CAD build for the part. Positions are in the model's coordinates, mm. Face numbers are marked on the shaded views. A direction names the side the tool comes from. Give positions to 0.01 mm unless a question says otherwise; leave off trailing zeros. Loops run counter-clockwise (first coordinate to the right, second up) from the corner with the lowest first, then second, coordinate; pieces in that order, holes last.
Item 1: Saw through at B-B on x = 27.5. Give the cut face in (y, z).
Item 2: Drop flat-ended pins along their axis: P1, Ø1, axis at x = 22, y = -55, coming from the +Z side; P2, Ø15.5, axis at y = -67.5, z = 73, coming from the -X side; P3, Ø17.5, axis at x = 43.5, y = -8.5, coming from the +Z side. Give the stop position or say it passes through.
Item 3: Which spindle directions (+Z, -Z, +X, -X, +Y, -Y) get a long thin tool onto all of the face, cutting with end or side? Do the marked faces 4, 5 and 6. Say none if no direction does.
Item 4: Mould opens along Z. For the marked faces 1, 2 and 3 say: released by +Z, released by -Z, zero draft, split by the parting line, or undercut.
Item 5: Probe probe 1 along Y at (x, z) = (-40, 5); probe 2 along X at (y, z) = (-91.5, 71.5); probe 3 along X at (y, z) = (-119, 47). List the from-to ranges inside material, lowest first.
Item 6: Saw through at C-C on y = 22. Give the cut face in (x, z), plus the area to 3 significant figures.
Item 7: Saw through at A-A on y = -64. Give the cut face in (x, z).
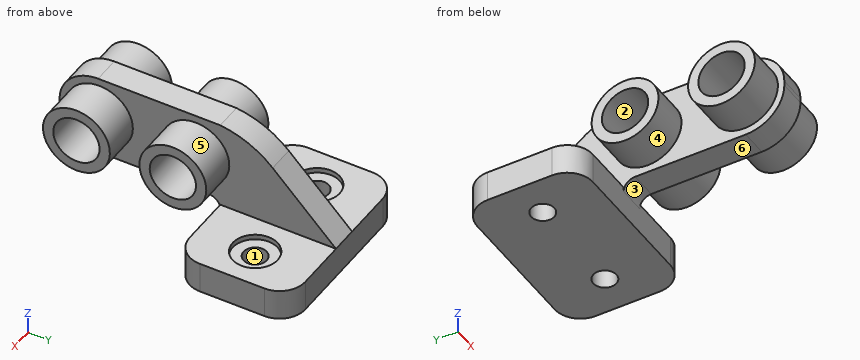
from build123d import *

# Parameters (mm, degrees)
CROQUIS2_W                   = 141
CROQUIS2_H                   = 90
SALIENTE_EXTRUIR1_DEPTH      = 24
REDONDEO1_R                  = 20
CROQUIS3_R                   = 17.5
CORTAR_EXTRUIR1_DEPTH        = 4
CROQUIS5_W                   = 21
CROQUIS5_H                   = 90
SALIENTE_EXTRUIR2_DEPTH      = 69
CHAFL_N1_SIZE                = 69
REDONDEO4_R                  = 69
CROQUIS10_W                  = 21
CROQUIS10_H                  = 63.589544636
SALIENTE_EXTRUIR6_DEPTH      = 125
REDONDEO6_R                  = 9
REDONDEO7_R                  = 30
SALIENTE_EXTRUIR8_DEPTH      = 30
SALIENTE_EXTRUIR8_DEPTH_BACK = 51
CROQUIS11_R                  = 26
CROQUIS15_R                  = 18
CORTAR_EXTRUIR3_DEPTH        = 224.315919719
CROQUIS16_R                  = 18
CORTAR_EXTRUIR4_DEPTH        = 224.315919719
CROQUIS17_R                  = 9
CORTAR_EXTRUIR5_DEPTH        = 30
CROQUIS18_R                  = 9
CORTAR_EXTRUIR6_DEPTH        = 30


with BuildPart() as part:
    # Croquis2 → Saliente-Extruir1 (new body)
    with BuildSketch(Plane.XY):
        Rectangle(CROQUIS2_W, CROQUIS2_H)
    extrude(amount=SALIENTE_EXTRUIR1_DEPTH)

    # Redondeo1
    redondeo1_edges = [part.edges().sort_by_distance(p)[0] for p in [
        (70.5, -45, 12),
        (-70.5, -45, 12),
        (-70.5, 45, 12),
        (70.5, 45, 12),
    ]]
    fillet(redondeo1_edges, radius=REDONDEO1_R)

    # Croquis3 → Cortar-Extruir1 (cut)
    with BuildSketch(Plane.XY.offset(24)):
        with Locations((-40.5, 0)):
            Circle(CROQUIS3_R)
        with Locations(Location((40.5, 0, 0), (0, 0, 180))):
            Circle(CROQUIS3_R)
    extrude(amount=-CORTAR_EXTRUIR1_DEPTH, mode=Mode.SUBTRACT)

    # Croquis5 → Saliente-Extruir2 (add)
    with BuildSketch(Plane.XY.offset(24)):
        Rectangle(CROQUIS5_W, CROQUIS5_H)
    extrude(amount=SALIENTE_EXTRUIR2_DEPTH)

    # Chaflán1
    chafl_n1_edges = [part.edges().sort_by_distance(p)[0] for p in [
        (0, 45, 93),
    ]]
    chamfer(chafl_n1_edges, length=CHAFL_N1_SIZE)

    # Redondeo4
    # the kernel refuses this fillet: 69 mm, written as the material it takes off along each edge
    with BuildSketch(Plane(origin=(-80.285016103, -24, 93), x_dir=(0, 0.7071067811865477, -0.7071067811865474), z_dir=(1, 0, 0))) as redondeo4_piece_1:
        with BuildLine():
            CenterArc((27.914006441, -69), REDONDEO4_R, 90, 38.298408264)
            Line((-14.849242405, -14.849242405), (-15.704507382, -13.766227253))
            ThreePointArc((-15.704507382, -13.766227253), (-8.40042856, -6.448813844), (-0.975807358, 0.975807358))
            Line((-0.975807358, 0.975807358), (0, 1.38))
            Line((0, 1.38), (27.914006441, 1.38))
            Line((27.914006441, 1.38), (27.914006441, 0))
        make_face()
    extrude(amount=160.570032206, mode=Mode.SUBTRACT)

    # Croquis10 → Saliente-Extruir6 (add)
    with BuildSketch(Plane(origin=(0, -45, 0), x_dir=(-1, 0, 0), z_dir=(0, -1, 0))):
        with Locations((0, -61.205227682)):
            Rectangle(CROQUIS10_W, CROQUIS10_H)
    extrude(amount=SALIENTE_EXTRUIR6_DEPTH)

    # Redondeo6
    # the kernel refuses this fillet: 9 mm, written as the material it adds along each edge
    with BuildSketch(Plane(origin=(-10.5, -45, 29.410455364), x_dir=(0, 0, -1), z_dir=(1, 0, 0))) as redondeo6_piece_1:
        with BuildLine():
            CenterArc((REDONDEO6_R, -REDONDEO6_R), REDONDEO6_R, 90, 90)
            Line((0, -REDONDEO6_R), (0, 0))
            Line((0, 0), (REDONDEO6_R, 0))
        make_face()
    extrude(amount=21)

    # Redondeo7
    redondeo7_edges = [part.edges().sort_by_distance(p)[0] for p in [
        (0, -170, 93),
        (0, -170, 29.410455364),
    ]]
    fillet(redondeo7_edges, radius=REDONDEO7_R)

    # Croquis11 → Saliente-Extruir8 (add, two sides: drawn at the far end of the back side and taken through both)
    with BuildSketch(Plane(origin=(10.5, 0, 0), x_dir=(0, 0, -1), z_dir=(1, 0, 0)).offset(-SALIENTE_EXTRUIR8_DEPTH_BACK)):
        with Locations((-61.205227682, -64)):
            Circle(CROQUIS11_R)
        with Locations((-61.205227682, -139)):
            Circle(CROQUIS11_R)
    extrude(amount=SALIENTE_EXTRUIR8_DEPTH + SALIENTE_EXTRUIR8_DEPTH_BACK)

    # Croquis15 → Cortar-Extruir3 (cut, through all)
    with BuildSketch(Plane(origin=(40.5, 0, 0), x_dir=(0, 0, -1), z_dir=(1, 0, 0))):
        with Locations((-61.205227682, -64)):
            Circle(CROQUIS15_R)
    extrude(amount=-CORTAR_EXTRUIR3_DEPTH, mode=Mode.SUBTRACT)

    # Croquis16 → Cortar-Extruir4 (cut, through all)
    with BuildSketch(Plane(origin=(40.5, 0, 0), x_dir=(0, 0, -1), z_dir=(1, 0, 0))):
        with Locations((-61.205227682, -139)):
            Circle(CROQUIS16_R)
    extrude(amount=-CORTAR_EXTRUIR4_DEPTH, mode=Mode.SUBTRACT)

    # Croquis17 → Cortar-Extruir5 (cut)
    with BuildSketch(Plane.XY.offset(20)):
        with Locations((40.5, 0)):
            Circle(CROQUIS17_R)
    extrude(amount=-CORTAR_EXTRUIR5_DEPTH, mode=Mode.SUBTRACT)

    # Croquis18 → Cortar-Extruir6 (cut)
    with BuildSketch(Plane.XY.offset(20)):
        with Locations((-40.5, 0)):
            Circle(CROQUIS18_R)
    extrude(amount=-CORTAR_EXTRUIR6_DEPTH, mode=Mode.SUBTRACT)


solid = part.part
Results below:
1. outline: circle Ø52 at (-139, 61.21); circle Ø52 at (-64, 61.21); (-45, 0) - (45, 0) - (45, 24) - (11.72, 24) - (11.72, 20) - (-11.72, 20) - (-11.72, 24) - (-45, 24) - close; hole circle Ø36 at (-139, 61.21); hole circle Ø36 at (-64, 61.21)
2. P1: stops at z = 85.78
2. P2: stops at x = -40.5
2. P3: stops at z = 24
3. face 4: -X
3. face 5: +X
3. face 6: -Z, +X, -X, -Y
4. face 1: zero draft
4. face 2: undercut
4. face 3: released by -Z
5. probe 1: y = -45 to -8.99, 8.99 to 45
5. probe 2: x = -10.5 to 10.5
5. probe 3: x = -40.5 to 40.5
6. outline: (-70.5, 0) - (70.5, 0) - (70.5, 24) - (10.5, 24) - (10.5, 47) - (-10.5, 47) - (-10.5, 24) - (-70.5, 24) - close
6. area: 3,870 mm2
7. outline: (-40.5, 35.21) - (-10.5, 35.21) - (-10.5, 29.41) - (10.5, 29.41) - (10.5, 35.21) - (40.5, 35.21) - (40.5, 43.21) - (-40.5, 43.21) - close; (-40.5, 79.21) - (40.5, 79.21) - (40.5, 87.21) - (10.5, 87.21) - (10.5, 93) - (-10.5, 93) - (-10.5, 87.21) - (-40.5, 87.21) - close
